Geometry check sheet. Reference: the model listing, model coordinates, mm. Face numbers are marked on the shaded views. Give positions to 0.01 mm unless a question says otherwise; leave off trailing zeros. Loops run counter-clockwise (first coordinate to the right, second up) from the corner with the lowest first, then second, coordinate; pieces in that order, holes last. Notation, with made-up numbers: (28.5, 29.25) - (78.5, 29.25) arc R23 cw to (78.5, 44.25) - close; hole circle Ø1 at (64, -32.75). An arc over 180 degrees is marked (long way). Write item = value, one per line. Start each with the question number.
from build123d import *

# Parameters (mm, degrees)
F0_W     = 20
F0_H     = 20
F1_DEPTH = 10
F3_D     = 10
F4_R     = 5


with BuildPart() as f1:
    # F0 (on Top) → F1 (new body)
    with BuildSketch(Plane.XY):
        Rectangle(F0_W, F0_H)
    extrude(amount=F1_DEPTH)

    # F3 (through all)
    with Locations(Plane.XY.offset(10)):
        with Locations((0, 0)):
            Hole(F3_D / 2)

    # F4
    f4_edges = [f1.edges().sort_by_distance(p)[0] for p in [
        (10, 10, 5),
    ]]
    fillet(f4_edges, radius=F4_R)


solid = f1.part
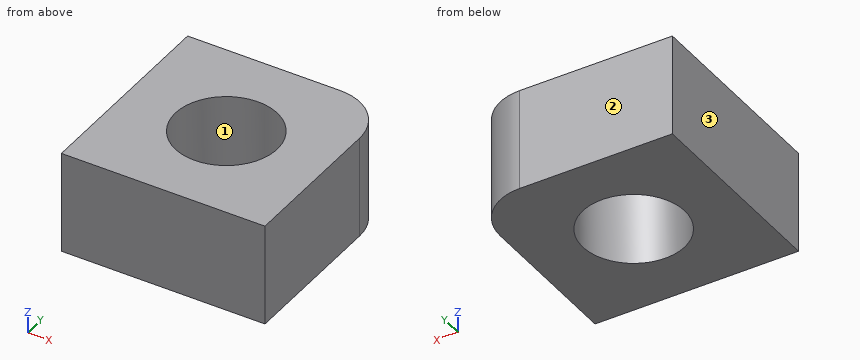
1) Cross-section at C-C on z = 3. Enter the section's corners in (x, y).
2) Material ranges on line 1 along Y through (x, z) = (0, 3.5); line 2 along X through (y, z) = (-0.5, 6.5); line 3 along X through (y, z) = (4.5, 3), recorded low to high.
3) Cross-section at A-A on y = 0. Enter the section's corners in (x, z).
4) Release check for a two-part mould opening along Y. For the marked faces 1, 2 and 3 record: pulls with the +Y half, pulls with the -Y half, needs draft (parallel to the pull), parting line crosses it, or undercut.
5) Cross-section at D-D on y = 7. Enter the section's corners in (x, z).
Checked values:
q1.outline = (-10, -10) - (10, -10) - (10, 5) arc R5 ccw to (5, 10) - (-10, 10) - close; hole circle Ø10 at (0, 0)
q2.line_1 = -10 to -5, 5 to 10
q2.line_2 = -10 to -4.97, 4.97 to 10
q2.line_3 = -10 to -2.18, 2.18 to 10
q3.outline = (-10, 0) - (-5, 0) - (-5, 10) - (-10, 10) - close; (5, 0) - (10, 0) - (10, 10) - (5, 10) - close
q4.face_1 = undercut
q4.face_2 = pulls with the +Y half
q4.face_3 = needs draft
q5.outline = (-10, 0) - (9.58, 0) - (9.58, 10) - (-10, 10) - close
